Read the model definition and answer for the solid it produces. Units are mm, in the model's axes. Face numbers are marked on the shaded views. A direction names the side the tool comes from. Round coordinates to 2 decimals unless told otherwise and drop trailing zeros. Write each loop counter-clockwise with the first axis right and the second up, starting at its lowest first coordinate (ties: lowest second). Pieces come first, ordered by that corner, then holes. Notation, with made-up numbers: (73.5, -17) - (128.5, -17) arc R15 ccw to (128.5, -9) - close; hole circle Ø2 at (69.5, -21). An arc over 180 degrees is marked (long way). Use one line per item in the form item = value. Start each with the question number.
1) The part is cut by section B-B, the plane x = 3. Give the vertices of the cut face in (y, z) (3 decimals), plus the area to 3 significant figures.
2) Consider line 1 along X through (y, z) = (-2.75, 10); line 2 along X through (y, z) = (0.25, -1.75); line 3 along Y through (x, z) = (-3, -4.5). Determine where each line is inside the solid, lowest interval first. Write a range as from..to.
3) For a pull along X with two mould halves and no side action, classify the marked faces 6, 7 and 8 as released by +X, released by -X, zero draft, split by the parting line, or undercut.
4) For the marked faces 1, 2, 3, 4 and 5, determine the directions among +Z, -Z, +X, -X, +Y, -Y from which every point of the face is accessible in a straight line to the end or side of a thin tool.
5) Each of these flat-tipped pins is pushed along its axis until it touches: pin 1 (1.5 mm diameter, centred on x = 2.5, y = -1, fed in from +Z) (3 decimals); pin 2 (3 mm diameter, centred on y = -6, z = -5.5, fed in from -X); pin 3 (2.5 mm diameter, centred on y = 0.5, z = -12.5, fed in from -X). Where does it stop, or does it pass through?
6) The part is cut by section A-A, the plane z = 10. Give the vertices of the cut face in (x, y).
7) The part is cut by section D-D, the plane z = 4.25. Give the vertices of the cut face in (x, y), plus the area to 3 significant figures.
from build123d import *

# Parameters (mm, degrees)
BOSS_EXTRUDE1_DEPTH = 14.835
CUT_EXTRUDE1_REACH  = 37.321
SKETCH4_R           = 1.65
SKETCH4_3_W         = 6
SKETCH4_3_H         = 5
SKETCH4_3_R         = 1.65
CUT_EXTRUDE3_DEPTH  = 7
CUT_EXTRUDE2_REACH  = 26.619
SKETCH5_R           = 3.75
SKETCH6_W           = 4
SKETCH6_H           = 6
BOSS_EXTRUDE2_DEPTH = 29.67


with BuildPart() as part:
    # Sketch3 → Boss-Extrude1 (new, symmetric)
    with BuildSketch(Plane.XY):
        Polygon((-19, 2.5), (-10.339745962, -2.5), (19, -2.5), (19, 2.5), align=None)
    extrude(amount=BOSS_EXTRUDE1_DEPTH, both=True)

    # Sketch4 → Cut-Extrude1 (cut, up to next)
    with BuildSketch(Plane.XY.offset(14.835), mode=Mode.PRIVATE) as cut_extrude1_sk1:
        with Locations((3, 0)):
            Circle(SKETCH4_R)
    cut_extrude1_tool1 = extrude(cut_extrude1_sk1.sketch, amount=-CUT_EXTRUDE1_REACH, mode=Mode.PRIVATE) & part.part
    add(cut_extrude1_tool1.solids().sort_by_distance((3, 0, 14.835))[0], mode=Mode.SUBTRACT)

    # Sketch4<3> → Cut-Extrude3 (cut)
    with BuildSketch(Plane.XY.offset(14.835)):
        with Locations((3, 0)):
            Rectangle(SKETCH4_3_W, SKETCH4_3_H)
        with Locations((3, 0)):
            Circle(SKETCH4_3_R, mode=Mode.SUBTRACT)
    cut_extrude3 = extrude(amount=-CUT_EXTRUDE3_DEPTH, mode=Mode.SUBTRACT)

    # Mirror1: Cut-Extrude3 across plane
    add(cut_extrude3.mirror(Plane.XY), mode=Mode.SUBTRACT)

    # Sketch5 → Cut-Extrude2 (cut, up to next)
    with BuildSketch(Plane(origin=(0, 2.5, 0), x_dir=(1, 0, 0), z_dir=(0, 1, 0)), mode=Mode.PRIVATE) as cut_extrude2_sk1:
        with Locations(Location((3, 0, 0), (0, 0, 270))):
            Circle(SKETCH5_R)
    cut_extrude2_tool1 = extrude(cut_extrude2_sk1.sketch, amount=-CUT_EXTRUDE2_REACH, mode=Mode.PRIVATE) & part.part
    add(cut_extrude2_tool1.solids().sort_by_distance((3, 2.5, 0))[0], mode=Mode.SUBTRACT)

    # Sketch6 → Boss-Extrude2 (add)
    with BuildSketch(Plane.XY.offset(14.835)):
        with Locations((17, -5.5)):
            Rectangle(SKETCH6_W, SKETCH6_H)
    extrude(amount=-BOSS_EXTRUDE2_DEPTH)


solid = part.part
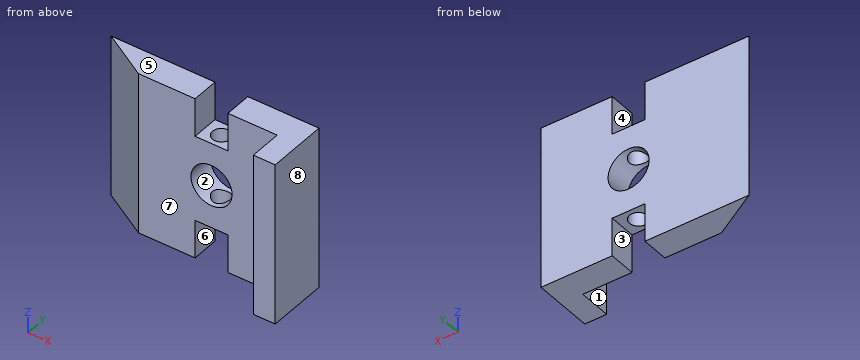
Geometry results:
q1.outline = (-2.5, -7.835) - (-1.65, -7.835) - (-1.65, -3.75) - (-2.5, -3.75) - close; (-2.5, 3.75) - (-1.65, 3.75) - (-1.65, 7.835) - (-2.5, 7.835) - close; (1.65, -7.835) - (2.5, -7.835) - (2.5, -3.75) - (1.65, -3.75) - close; (1.65, 3.75) - (2.5, 3.75) - (2.5, 7.835) - (1.65, 7.835) - close
q1.area = 13.9 mm2
q2.line_1 = 15..19
q2.line_2 = -15.1..-0.32, 6.32..19
q2.line_3 = -2.5..2.5
q3.face_6 = undercut
q3.face_7 = zero draft
q3.face_8 = released by +X
q4.face_1 = +Z, -Z, -X, -Y
q4.face_2 = +Y, -Y
q4.face_3 = -Z, +Y, -Y
q4.face_4 = +Z, +Y, -Y
q4.face_5 = +Z, +X, -X, +Y, -Y
q5.pin_1 = 7.835
q5.pin_2 = 15
q5.pin_3 = -17.7
q6.outline = (-19, 2.5) - (-10.34, -2.5) - (0, -2.5) - (0, 2.5) - close; (6, -2.5) - (15, -2.5) - (15, -8.5) - (19, -8.5) - (19, 2.5) - (6, 2.5) - close
q7.outline = (-19, 2.5) - (-10.34, -2.5) - (15, -2.5) - (15, -8.5) - (19, -8.5) - (19, 2.5) - close; hole circle Ø3.3 at (3, 0)
q7.area = 184 mm2
